Input: part model. Units: mm. Frame: model coordinates. Round coordinates to 2 decimals unless told otherwise and drop trailing zeros. Loops run counter-clockwise (first coordinate to the right, second up) from the corner with the lowest first, then second, coordinate; pieces in that order, holes last. Notation, with made-up numbers: M 51.25,2.25 L 73.25,2.25 A31 ccw 73.25,38.25 Z; hole C -18,50 d4. An arc over 180 degrees is marked long. Put each result on its own line as item: value. Start each with the question number.
1) Draft query along X for faces 1 (the face through (-19.32, -1.57, -16.05)), 2 (the face through (-3, -3.175, -62)). Return one class per face: +X half, -X half, draft (parallel to the pull), parting line (faces both ways), or undercut.
2) Section D-D on x = -78. Output: boundary loops of the cut face in (y, z) (3 decimals).
3) Line query: probe 1 along X at (y, z) = (-2.1, 181.5); probe 2 along X at (y, z) = (-2.3, 10); probe 3 along Z at (x, y) = (44.5, -2.5). Output: solid intervals per line, ascending.
4) Section A-A on x = 0. Output: boundary loops of the cut face in (y, z) (3 decimals).
5) Section C-C on y = -1. Output: boundary loops of the cut face in (x, z), plus the area to 3 significant figures.
6) Section B-B on z = 32. Output: boundary loops of the cut face in (x, y) (3 decimals).
from build123d import *

# Parameters (mm, degrees)
SKETCH1_W          = 368.3
SKETCH1_H          = 520.7
BASE_FLANGE1_DEPTH = 3.175
SKETCH6_W          = 203.2
SKETCH6_H          = 184.912
CUT_EXTRUDE1_DEPTH = 319.909745265
SKETCH7_R          = 31.75
CUT_EXTRUDE2_DEPTH = 319.909745265


# Sheet-metal steps are written as plain solids
with BuildPart() as part:
    # Sketch1 → Base-Flange1 (new body)
    with BuildSketch(Plane(origin=(0, 0, 0), x_dir=(1, 0, 0), z_dir=(0, 1, 0))):
        Rectangle(SKETCH1_W, SKETCH1_H)
    extrude(amount=-BASE_FLANGE1_DEPTH)

    # Sketch6 → Cut-Extrude1 (cut, through all)
    with BuildSketch(Plane(origin=(0, 0, 0), x_dir=(1, 0, 0), z_dir=(0, 1, 0))):
        with Locations((0, -260.35)):
            Rectangle(SKETCH6_W, SKETCH6_H)
    extrude(amount=-CUT_EXTRUDE1_DEPTH, mode=Mode.SUBTRACT)

    # Sketch7 → Cut-Extrude2 (cut, through all)
    with BuildSketch(Plane(origin=(0, 0, 0), x_dir=(1, 0, 0), z_dir=(0, 1, 0))):
        with Locations(Location((0, -9.144, 0), (0, 0, 270))):
            Circle(SKETCH7_R)
    extrude(amount=-CUT_EXTRUDE2_DEPTH, mode=Mode.SUBTRACT)


solid = part.part
Geometry results:
1. face 1: undercut
1. face 2: draft
2. outline: M -3.175,-260.35 L 0,-260.35 L 0,167.894 L -3.175,167.894 Z
3. probe 1: x = -184.15 to -101.6, 101.6 to 184.15
3. probe 2: x = -184.15 to -31.74, 31.74 to 184.15
3. probe 3: z = -260.35 to 167.89
4. outline: M -3.175,-260.35 L 0,-260.35 L 0,-22.606 L -3.175,-22.606 Z; M -3.175,40.894 L 0,40.894 L 0,167.894 L -3.175,167.894 Z
5. outline: M -184.15,-260.35 L 184.15,-260.35 L 184.15,260.35 L 101.6,260.35 L 101.6,167.89 L -101.6,167.89 L -101.6,260.35 L -184.15,260.35 Z; hole C 0,9.14 d63.5
5. area: 170,000 mm²
6. outline: M -184.15,-3.175 L -22.038,-3.175 L -22.038,0 L -184.15,0 Z; M 22.038,-3.175 L 184.15,-3.175 L 184.15,0 L 22.038,0 Z
